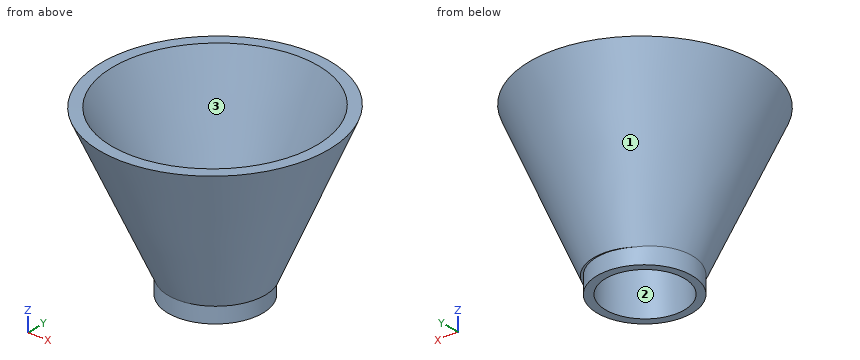
from build123d import *

# Parameters (mm, degrees)
F2_R     = 20.9843875465
F3_DEPTH = 25.4
F5_R     = 17.4817395379
F6_DEPTH = 25.4


with BuildPart() as f1:
    # F0 (on Front) → F1 (revolve)
    with BuildSketch(Plane.XZ):
        Polygon((-32.9396761954, 21.1004912853), (-54.5175522566, 21.1004912853), (-54.3266013265, 7.5427088886), (-32.9396761954, 7.5427088886), (-4.8693441786, 74.185885489), (-10.025119409, 74.185885489), align=None)
    revolve(axis=Axis((-54.4220767915, 0, 14.321600087), (-0.0140828336, 0, 0.999900832)))

    # F2 (on Top) → F3 (join)
    with BuildSketch(Plane.XY):
        with Locations((-55.1074631512, 0)):
            Circle(F2_R)
    extrude(amount=F3_DEPTH)

    # F5 (on face) → F6 (cut)
    with BuildSketch(Plane(origin=(0, 0, 0), x_dir=(1, 0, 0), z_dir=(0, 0, -1))):
        with Locations((-55.2984140813, 0)):
            Circle(F5_R)
    extrude(amount=-F6_DEPTH, mode=Mode.SUBTRACT)


solid = f1.part
CAD build for the part. Positions are in the model's coordinates, mm. Face numbers are marked on the shaded views. Give positions to 0.01 mm unless a question says otherwise; leave off trailing zeros. Answer in a Markdown table with one row per item. Add a question column.
Item 1: Mould opens along X. For the marked faces 1, 2 and 3 say: +X half, -X half, draft (parallel to the pull), parting line (faces both ways), or undercut.
Item 2: Probe probe 1 along X at (y, z) = (0, 7.25); probe 2 along Y at (x, z) = (-57.5, 48.5); probe 3 along X at (y, z) = (0, 17.75). List the from-to ranges inside material, lowest first.
Item 3: Drop flat-ended pins along their axis: P1, Ø8, axis at x = -64, z = 15.5, coming from the -Y side; P2, Ø8, axis at y = 28.5, z = 50.5, coming from the -X side; P3, Ø12, axis at y = -13, z = 28, coming from the +X side. Give the stop position or say it passes through.
Reply:
| question | item | result |
|---|---|---|
| 1 | face 1 | parting line |
| 1 | face 2 | undercut |
| 1 | face 3 | undercut |
| 2 | probe 1 | x = -76.09 to -72.78, -37.82 to -34.12 |
| 2 | probe 2 | y = -39.38 to -33.92, 33.92 to 39.38 |
| 2 | probe 3 | x = -80.62 to -72.78, -37.82 to -28.64 |
| 3 | P1 | stops at y = -25.48 |
| 3 | P2 | stops at x = -87.97 |
| 3 | P3 | stops at x = -23.68 |
